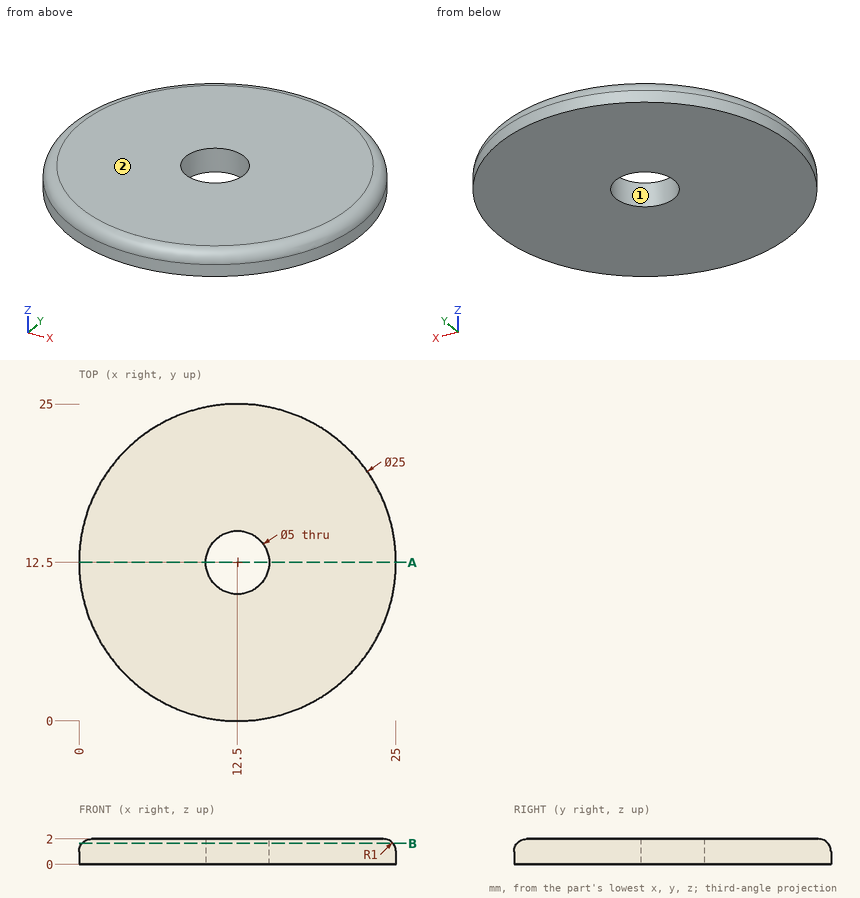
Design review of the part shown in the three views and the two pictorial views. Dimensions are in mm from the part's minimum x, y and z. Give positions to 0.01 mm unless a question says otherwise; leave off trailing zeros. Write each loop counter-clockwise with the first axis right and the second up, starting at its lowest first coordinate (ties: lowest second). Pieces come first, ordered by that corner, then holes.
Item 1: Take a section at B-B (z = 1.65). Give the boundary of the cut face in (x, y).
Item 2: Take a section at A-A (y = 12.5). Give the boundary of the cut face in (x, z).
Item 3: Insertion check: P1, Ø1, axis at y = 5, z = 1.5, coming from the -X side; P2, Ø4.5, axis at x = 12.5, y = 12.5, coming from the +Z side. Each pin has a flat end and moves straight along its axis. Give the tip position at first contact, or say it passes through.
Item 4: The part is to be moulded in two halves that separate along X. For the marked faces 1 and 2, say which applies: +X half, -X half, draft (parallel to the pull), parting line (faces both ways), or undercut.
Item 5: Wall thickness on probe 1 along Y at (x, z) = (12.5, 0.55); probe 2 along Y at (x, z) = (14.25, 1.2); probe 3 along Y at (x, z) = (4, 0.65): over which ranges is each line inside the solid? List them lowest first.
Established:
1. outline: circle Ø24.52 at (12.5, 12.5); hole circle Ø5 at (12.5, 12.5)
2. outline: (0, 0) - (10, 0) - (10, 2) - (1, 2) arc R1 ccw to (0, 1) - close; (15, 0) - (25, 0) - (25, 1) arc R1 ccw to (24, 2) - (15, 2) - close
3. P1: stops at x = 2.23
3. P2: passes through
4. face 1: undercut
4. face 2: draft
5. probe 1: y = 0 to 10, 15 to 25
5. probe 2: y = 0.14 to 10.71, 14.29 to 24.86
5. probe 3: y = 3.33 to 21.67
